Here's how the part is built. I have some questions about the finished solid (model axes, mm). Face numbers are marked on the shaded views. Round coordinates to 2 decimals unless told otherwise and drop trailing zeros. Loops run counter-clockwise (first coordinate to the right, second up) from the corner with the lowest first, then second, coordinate; pieces in that order, holes last. Notation, with made-up numbers: M -20.75,27.25 L 12.25,27.25 A10 ccw 12.25,45.25 Z; hole C 71.5,-8.5 d11. An arc over 180 degrees is marked long. Answer as a JSON object with one key per item and string values.
from build123d import *

# Parameters (mm, degrees)
SKETCH1_W           = 2768.6
SKETCH1_H           = 812.8
BOSS_EXTRUDE1_DEPTH = 177.8
SKETCH2_R           = 25.4
CUT_EXTRUDE1_DEPTH  = 831.342
SKETCH3_W           = 2644.359498688
SKETCH3_H           = 740.774814922
CUT_EXTRUDE2_DEPTH  = 166.37
CUT_EXTRUDE3_DEPTH  = 57.912
FILL_START          = 166.37
FILL_PATTERN1_DEPTH = 11.43
SCALE1_SCALE        = 0.5867


# Read off the part's stored shape, not the designer's step: Fill Pattern1
with BuildPart() as part:
    # Sketch1 → Boss-Extrude1 (new body)
    with BuildSketch(Plane(origin=(0, 0, 0), x_dir=(1, 0, 0), z_dir=(0, 1, 0))):
        Rectangle(SKETCH1_W, SKETCH1_H)
    extrude(amount=BOSS_EXTRUDE1_DEPTH)

    # Sketch2 → Cut-Extrude1 (cut)
    with BuildSketch(Plane.XY.offset(406.4)):
        with Locations((-1296.438284971, 103.124)):
            Circle(SKETCH2_R)
    extrude(amount=-CUT_EXTRUDE1_DEPTH, mode=Mode.SUBTRACT)

    # Sketch3 → Cut-Extrude2 (cut)
    with BuildSketch(Plane.XZ):
        Rectangle(SKETCH3_W, SKETCH3_H)
    extrude(amount=-CUT_EXTRUDE2_DEPTH, mode=Mode.SUBTRACT)

    # Sketch12 → Cut-Extrude3 (cut)
    with BuildSketch(Plane.XZ.offset(-166.37)):
        with BuildLine():
            Line((-897.344557037, 264.630737371), (-897.344557037, -215.907837093))
            ThreePointArc((-897.344557037, -215.907837093), (-978.253251545, -296.816531601), (-1059.161946053, -215.907837093))
            Line((-1059.161946053, -215.907837093), (-1059.161946053, 264.630737371))
            ThreePointArc((-1059.161946053, 264.630737371), (-978.253251545, 345.539431879), (-897.344557037, 264.630737371))
        make_face()
    extrude(amount=-CUT_EXTRUDE3_DEPTH, mode=Mode.SUBTRACT)

    # Fill Pattern1 outline → Fill Pattern1 (cut)
    with BuildSketch(Plane(origin=(0, 0, 0), x_dir=(1, 0, 0), z_dir=(0, 1, 0)).offset(FILL_START)):
        with BuildLine():
            ThreePointArc((-789.87554691, -264.630737371), (-708.966852402, -345.539431879), (-628.058157894, -264.630737371))
            Line((-628.058157894, -264.630737371), (-628.058157894, 215.907837093))
            ThreePointArc((-628.058157894, 215.907837093), (-708.966852402, 296.816531601), (-789.87554691, 215.907837093))
            Line((-789.87554691, 215.907837093), (-789.87554691, -264.630737371))
        make_face()
        with BuildLine():
            ThreePointArc((1095.129247093, -264.630737371), (1176.0379416, -345.539431879), (1256.946636108, -264.630737371))
            Line((1256.946636108, -264.630737371), (1256.946636108, 215.907837093))
            ThreePointArc((1256.946636108, 215.907837093), (1176.0379416, 296.816531601), (1095.129247093, 215.907837093))
            Line((1095.129247093, 215.907837093), (1095.129247093, -264.630737371))
        make_face()
        with BuildLine():
            ThreePointArc((825.842847949, -264.630737371), (906.751542457, -345.539431879), (987.660236965, -264.630737371))
            Line((987.660236965, -264.630737371), (987.660236965, 215.907837093))
            ThreePointArc((987.660236965, 215.907837093), (906.751542457, 296.816531601), (825.842847949, 215.907837093))
            Line((825.842847949, 215.907837093), (825.842847949, -264.630737371))
        make_face()
        with BuildLine():
            ThreePointArc((556.556448806, -264.630737371), (637.465143314, -345.539431879), (718.373837822, -264.630737371))
            Line((718.373837822, -264.630737371), (718.373837822, 215.907837093))
            ThreePointArc((718.373837822, 215.907837093), (637.465143314, 296.816531601), (556.556448806, 215.907837093))
            Line((556.556448806, 215.907837093), (556.556448806, -264.630737371))
        make_face()
        with BuildLine():
            ThreePointArc((287.270049663, -264.630737371), (368.178744171, -345.539431879), (449.087438678, -264.630737371))
            Line((449.087438678, -264.630737371), (449.087438678, 215.907837093))
            ThreePointArc((449.087438678, 215.907837093), (368.178744171, 296.816531601), (287.270049663, 215.907837093))
            Line((287.270049663, 215.907837093), (287.270049663, -264.630737371))
        make_face()
        with BuildLine():
            ThreePointArc((17.98365052, -264.630737371), (98.892345027, -345.539431879), (179.801039535, -264.630737371))
            Line((179.801039535, -264.630737371), (179.801039535, 215.907837093))
            ThreePointArc((179.801039535, 215.907837093), (98.892345027, 296.816531601), (17.98365052, 215.907837093))
            Line((17.98365052, 215.907837093), (17.98365052, -264.630737371))
        make_face()
        with BuildLine():
            ThreePointArc((-251.302748623, -264.630737371), (-170.394054116, -345.539431879), (-89.485359608, -264.630737371))
            Line((-89.485359608, -264.630737371), (-89.485359608, 215.907837093))
            ThreePointArc((-89.485359608, 215.907837093), (-170.394054116, 296.816531601), (-251.302748623, 215.907837093))
            Line((-251.302748623, 215.907837093), (-251.302748623, -264.630737371))
        make_face()
        with BuildLine():
            ThreePointArc((-520.589147766, -264.630737371), (-439.680453258, -345.539431879), (-358.771758751, -264.630737371))
            Line((-358.771758751, -264.630737371), (-358.771758751, 215.907837093))
            ThreePointArc((-358.771758751, 215.907837093), (-439.680453258, 296.816531601), (-520.589147766, 215.907837093))
            Line((-520.589147766, 215.907837093), (-520.589147766, -264.630737371))
        make_face()
    extrude(amount=FILL_PATTERN1_DEPTH, mode=Mode.SUBTRACT)


with BuildPart() as part_1:
    # Scale1: scaled about (-12.682340198, 104.835478071, -3.853275395)
    add(part.part.scale(SCALE1_SCALE).moved(Location((-5.241611204, 43.328503087, -1.592558721))))


solid = part_1.part
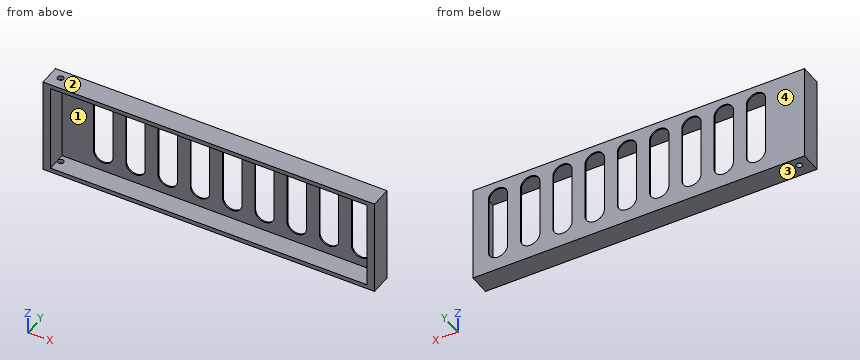
Item 1: Please list where these lines run through material, in increasing order: probe 1 along Z at (x, y) = (-180.5, 115); probe 2 along X at (y, z) = (126, -200.5); probe 3 along Y at (x, z) = (-657, -136.5). Write a range as from..to.
Resolved:
{"probe 1": "-240.03..-218.9, 215.71..236.84", "probe 2": "-817.41..-780.96, 770.48..806.93", "probe 3": "140.94..147.64"}
Item 2: I want a section at D-D, the plane x = 239. Please give me the cut outline in (y, z), then the cut area to 3 significant figures.
Resolved:
{"outline": "M 43.33,-240.03 L 147.64,-240.03 L 147.64,-166.43 L 140.94,-166.43 L 140.94,-218.9 L 43.33,-218.9 Z; M 43.33,215.71 L 140.94,215.71 L 140.94,191.83 L 147.64,191.83 L 147.64,236.84 L 43.33,236.84 Z", "area": "4,920 mm²"}
Item 3: I'm going to push a flat-ended pin straight in: pin 1 Ø2 at (x, z) = (310, -25.5) entering from -Y. Where does the tip first touch, or does it pass through?
Resolved:
{"pin 1": "y = 140.94"}
Item 4: If we mould it in two halves opening along Z, with no side actions, what happens to the marked faces 1, 2, 3 and 4? For each: pulls with the +Z half, pulls with the -Z half, needs draft (parallel to the pull), parting line crosses it, or undercut.
Resolved:
{"face 1": "undercut", "face 2": "pulls with the +Z half", "face 3": "pulls with the -Z half", "face 4": "needs draft"}
Item 5: I want a section at C-C, the plane z = -56. State how many separate pieces and enclosed holes the cut face has, then the cut area to 3 significant figures.
Resolved:
{"separate pieces": "10", "enclosed holes": "0", "area": "12,300 mm²"}
Item 6: I want a section at A-A, the plane y = 74.5. Please give me the cut outline in (x, z), then the cut area to 3 significant figures.
Resolved:
{"outline": "M -817.41,-240.03 L 806.93,-240.03 L 806.93,236.84 L -817.41,236.84 Z; hole M -780.96,-218.9 L 770.48,-218.9 L 770.48,215.71 L -780.96,215.71 Z", "area": "100,000 mm²"}
Item 7: I want a section at B-B, the plane x = -448.5. Please give me the cut outline in (y, z).
Resolved:
{"outline": "M 43.33,-240.03 L 147.64,-240.03 L 147.64,-167.09 L 140.94,-167.09 L 140.94,-218.9 L 43.33,-218.9 Z; M 43.33,215.71 L 140.94,215.71 L 140.94,192.49 L 147.64,192.49 L 147.64,236.84 L 43.33,236.84 Z"}
